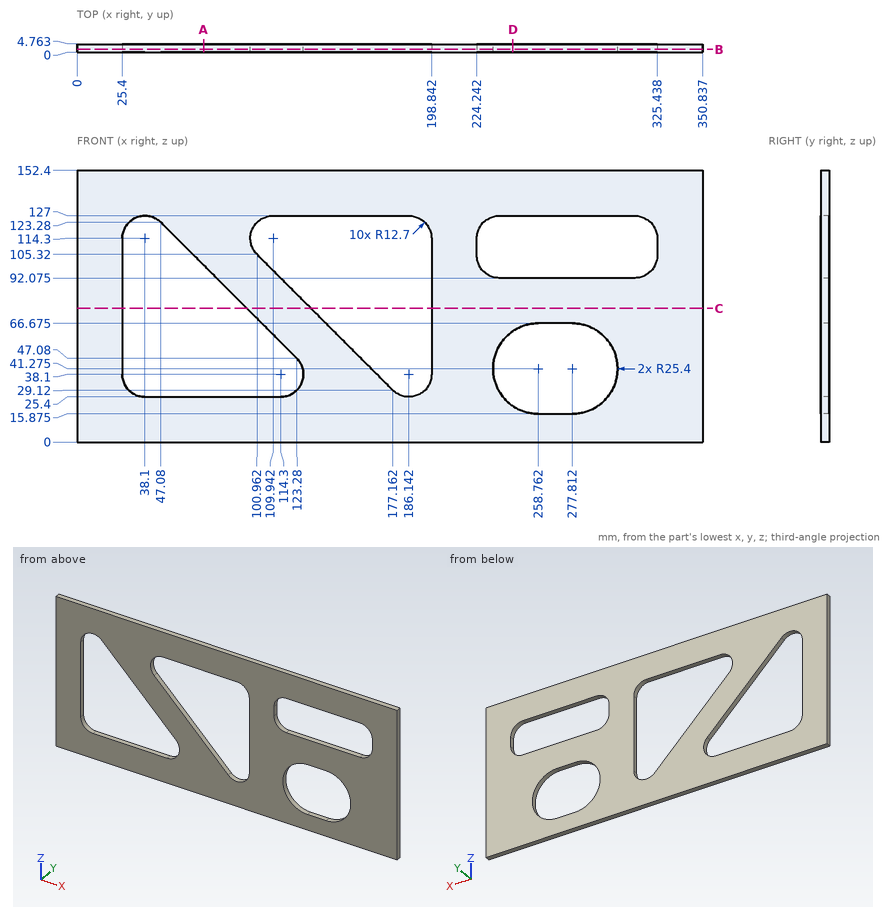
Here's the drawing with two shaded views (mm, measured from the low corner). I have some questions. Coordinates: 2 decimals unless noted, no trailing zeros. Order: outer loops, then holes, each group sorted by start corner. A loop starts at its lowest first (then second) coordinate and runs counter-clockwise, first axis right, second up.
Item 1: I need wall thicknesses on probe 1 along X at (y, z) = (3.9, 109) (1 decimal); probe 2 along X at (y, z) = (0.7, 84.5) (1 decimal); probe 3 along Z at (x, y) = (280.5, 1.95) (1 decimal). Which ranges of each line are inside material? Lowest first, please.
Response values:
probe 1: x = 0 to 25.4, 61.4 to 98.4, 198.8 to 224.2, 325.4 to 350.8
probe 2: x = 0 to 25.4, 85.9 to 121.8, 198.8 to 350.8
probe 3: z = 0 to 16, 66.5 to 92.1, 127 to 152.4
Item 2: If we section it at B-B, the plane y = 1.7: List the corners of the cut face in (x, z) for me (1 decimal).
Response values:
outline: (0, 0) - (350.8, 0) - (350.8, 152.4) - (0, 152.4) - close; hole (25.4, 38.1) arc R12.7 ccw to (38.1, 25.4) - (114.3, 25.4) arc R12.7 ccw to (123.3, 47.1) - (47.1, 123.3) arc R12.7 ccw to (25.4, 114.3) - close; hole (101, 105.3) - (177.2, 29.1) arc R12.7 ccw to (198.8, 38.1) - (198.8, 114.3) arc R12.7 ccw to (186.1, 127) - (109.9, 127) arc R12.7 ccw to start; hole (224.2, 104.8) arc R12.7 ccw to (236.9, 92.1) - (312.7, 92.1) arc R12.7 ccw to (325.4, 104.8) - (325.4, 114.3) arc R12.7 ccw to (312.7, 127) - (236.9, 127) arc R12.7 ccw to (224.2, 114.3) - close; hole (258.8, 15.9) - (277.8, 15.9) arc R25.4 ccw to (277.8, 66.7) - (258.8, 66.7) arc R25.4 ccw to start
Item 3: If we section it at A-A, the plane x = 71: List the corners of the cut face in (y, z) for me.
Response values:
outline: (0, 0) - (4.76, 0) - (4.76, 25.4) - (0, 25.4) - close; (0, 99.36) - (4.76, 99.36) - (4.76, 152.4) - (0, 152.4) - close
Item 4: If we section it at C-C, the plane z = 75: List the corners of the cut face in (x, y) for me, then the cut area to 3 significant figures.
Response values:
outline: (0, 0) - (25.4, 0) - (25.4, 4.76) - (0, 4.76) - close; (95.36, 0) - (131.28, 0) - (131.28, 4.76) - (95.36, 4.76) - close; (198.84, 0) - (350.84, 0) - (350.84, 4.76) - (198.84, 4.76) - close
area: 1,020 mm2
Item 5: If we section it at D-D, the plane x = 244.5: List the corners of the cut face in (y, z) for me (1 decimal).
Response values:
outline: (0, 0) - (4.8, 0) - (4.8, 20.3) - (0, 20.3) - close; (0, 62.3) - (4.8, 62.3) - (4.8, 92.1) - (0, 92.1) - close; (0, 127) - (4.8, 127) - (4.8, 152.4) - (0, 152.4) - close
